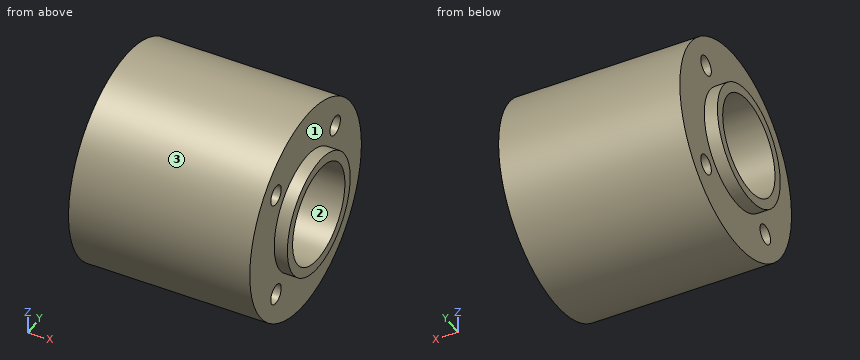
from build123d import *

# Parameters (mm, degrees)
SKETCH2_R          = 1.5
CUT_EXTRUDE1_DEPTH = 30.5
CIRPATTERN1_COUNT  = 4
SCALE1_SCALE       = 1.7


with BuildPart() as part:
    # Sketch1 → Revolve1 (revolve)
    with BuildSketch(Plane.XY):
        Polygon((0, 7.5), (0, 9), (2, 9), (2, 16), (29.5, 16), (29.5, 9), (31.5, 9), (31.5, 7.5), align=None)
    revolve(axis=Axis((0, 0, 0), (1, 0, 0)))

    # Sketch2 → Cut-Extrude1 (cut, through all)
    with BuildSketch(Plane.ZY.offset(-2)):
        with Locations((8.485281374, 8.485281374)):
            Circle(SKETCH2_R)
    cut_extrude1 = extrude(amount=-CUT_EXTRUDE1_DEPTH, mode=Mode.SUBTRACT)

    # CirPattern1: Cut-Extrude1 ×4 about axis
    cirpattern1_axis = Axis((0, 0, 0), (1, 0, 0))
    for i in range(1, CIRPATTERN1_COUNT):
        add(cut_extrude1.rotate(cirpattern1_axis, i * 360 / CIRPATTERN1_COUNT), mode=Mode.SUBTRACT)


with BuildPart() as part_1:
    # Scale1: scaled about (15.75, 0, 0)
    add(part.part.scale(SCALE1_SCALE).moved(Location((-11.025, 0, 0))))


solid = part_1.part
Verification items for the finished model (mm, model axes). Face numbers are marked on the shaded views. Give positions to 0.01 mm unless a question says otherwise; leave off trailing zeros. Write each loop counter-clockwise with the first axis right and the second up, starting at its lowest first coordinate (ties: lowest second). Pieces come first, ordered by that corner, then holes.
(1) Material ranges on line 1 (Z direction, x = -2.5, y = 13.5); line 2 (Z direction, x = -0.5, y = -15.5); line 3 (Y direction, x = 31, z = 13), recorded low to high.
(2) Mould release check, pull along Z, two halves, no side actions. Record for the marked faces 1, 2 and 3: +Z half, -Z half, draft (parallel to the pull), parting line (faces both ways), or undercut.
(3) Cross-section at A-A (y = 0). Enter the section's corners in (x, z) (3 decimals).
(4) Cross-section at D-D (x = 22.5). Enter the section's corners in (y, z).
(5) Cross-section at C-C (z = -13.5). Enter the section's corners in (x, y) (3 decimals), plus the area to 3 significant figures.
(6) Gauge pin test, flat ends, axial feed: pin 1 (2 mm diameter, centred on x = 16.5, z = -21.5, fed in from -Y); pin 2 (4 mm diameter, centred on x = 1, y = 2.5, fed in from +Z); pin 3 (6 mm diameter, centred on y = -14.42, z = -14.42, fed in from +X) (3 decimals). Record the tip position at first contact, or that the pin passes through.
Worked out:
1. line 1: z = -23.61 to -16.8, -12.05 to 12.05, 16.8 to 23.61
1. line 2: z = -22.35 to -16.74, -12.11 to 12.11, 16.74 to 22.35
1. line 3: y = -23.89 to -16.54, -12.31 to 12.31, 16.54 to 23.89
2. face 1: draft
2. face 2: undercut
2. face 3: parting line
3. outline: (-11.025, -15.3) - (-7.625, -15.3) - (-7.625, -27.2) - (39.125, -27.2) - (39.125, -15.3) - (42.525, -15.3) - (42.525, -12.75) - (-11.025, -12.75) - close; (-11.025, 12.75) - (42.525, 12.75) - (42.525, 15.3) - (39.125, 15.3) - (39.125, 27.2) - (-7.625, 27.2) - (-7.625, 15.3) - (-11.025, 15.3) - close
4. outline: circle Ø54.4 at (0, 0); hole circle Ø5.1 at (-14.42, -14.42); hole circle Ø5.1 at (-14.42, 14.42); hole circle Ø25.5 at (0, 0); hole circle Ø5.1 at (14.42, -14.42); hole circle Ø5.1 at (14.42, 14.42)
5. outline: (-11.025, -7.2) - (-7.625, -7.2) - (-7.625, -12.049) - (39.125, -12.049) - (39.125, -7.2) - (42.525, -7.2) - (42.525, 7.2) - (39.125, 7.2) - (39.125, 12.049) - (-7.625, 12.049) - (-7.625, 7.2) - (-11.025, 7.2) - close; (-7.625, -23.613) - (39.125, -23.613) - (39.125, -16.801) - (-7.625, -16.801) - close; (-7.625, 16.801) - (39.125, 16.801) - (39.125, 23.613) - (-7.625, 23.613) - close
5. area: 1,860 mm2
6. pin 1: stops at y = -17.88
6. pin 2: stops at z = 27.2
6. pin 3: stops at x = 39.125
